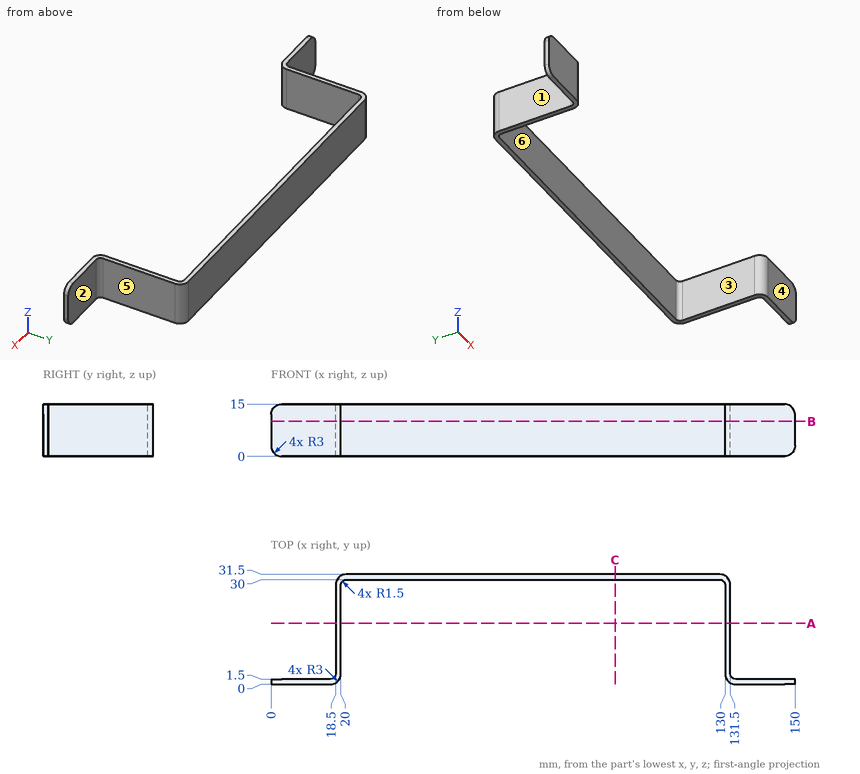
Drawing for the job (mm, zero at the part's lowest x, y, z). A direction names the side the tool comes from. Give positions to 0.01 mm unless a question says otherwise; leave off trailing zeros. Write each loop counter-clockwise with the first axis right and the second up, starting at its lowest first coordinate (ties: lowest second). Pieces come first, ordered by that corner, then holes. Notation, with made-up numbers: M 48.25,78.25 L 80.25,78.25 A14 cw 80.25,87.25 Z; hole C -12,-4 d4. An arc over 180 degrees is marked long. Return JSON: item names as keys, results as strings. Group by question number.
(1) Flat gauge pins, fed straight in: pin 1 Ø4.5 at (x, z) = (144.5, 10) entering from +Y; pin 2 Ø4.5 at (y, z) = (22, 8) entering from +X; pin 3 Ø1.5 at (x, y) = (133.5, 7.5) entering from +Z. Where does each tip first touch, or does it go through?
(2) Band-saw the part on C-C (x = 98.5). Give the cut face in (y, z).
(3) Mould opens along X. For the marked faces 4, 5 and 6 say: pulls with the +X half, pulls with the -X half, needs draft (parallel to the pull), parting line crosses it, or undercut.
(4) Drill centre lines: L1, parallel to X at y = 20, z = 9.75; L2, parallel to Y at x = 25, z = 4.25; L3, parallel to Y at x = 139.5, z = 4.75. Where is each one in solid material? Low to high. Write a range as [from, to].
(5) Band-saw the part on B-B (z = 10). Give the cut face in (x, y).
(6) 3-axis set-ups, long thin cutter, end or side, ignore diameter. For the marked faces 1, 2 and 3: which of +Z, -Z, +X, -X, +Y, -Y reach the whole face in a straight line?
(7) Band-saw the part on A-A (y = 17.5). Give the cut face in (x, z).
Entries:
{
 "1": {"pin 1": "stops at y = 1.5", "pin 2": "stops at x = 131.5", "pin 3": "passes through"},
 "2": {"outline": "M 30,0 L 31.5,0 L 31.5,15 L 30,15 Z"},
 "3": {"face 4": "needs draft", "face 5": "pulls with the +X half", "face 6": "undercut"},
 "4": {"L1": "x = [18.5, 20], [130, 131.5]", "L2": "y = [30, 31.5]", "L3": "y = [0, 1.5]"},
 "5": {"outline": "M 0,0 L 17,0 A3 ccw 20,3 L 20,28.5 A1.5 cw 21.5,30 L 128.5,30 A1.5 cw 130,28.5 L 130,3 A3 ccw 133,0 L 150,0 L 150,1.5 L 133,1.5 A1.5 cw 131.5,3 L 131.5,28.5 A3 ccw 128.5,31.5 L 21.5,31.5 A3 ccw 18.5,28.5 L 18.5,3 A1.5 cw 17,1.5 L 0,1.5 Z"},
 "6": {"face 1": "+Z, -Z, -X, +Y", "face 2": "+Z, -Z, +X, +Y", "face 3": "+Z, -Z, -Y"},
 "7": {"outline": "M 18.5,0 L 20,0 L 20,15 L 18.5,15 Z; M 130,0 L 131.5,0 L 131.5,15 L 130,15 Z"}
}
